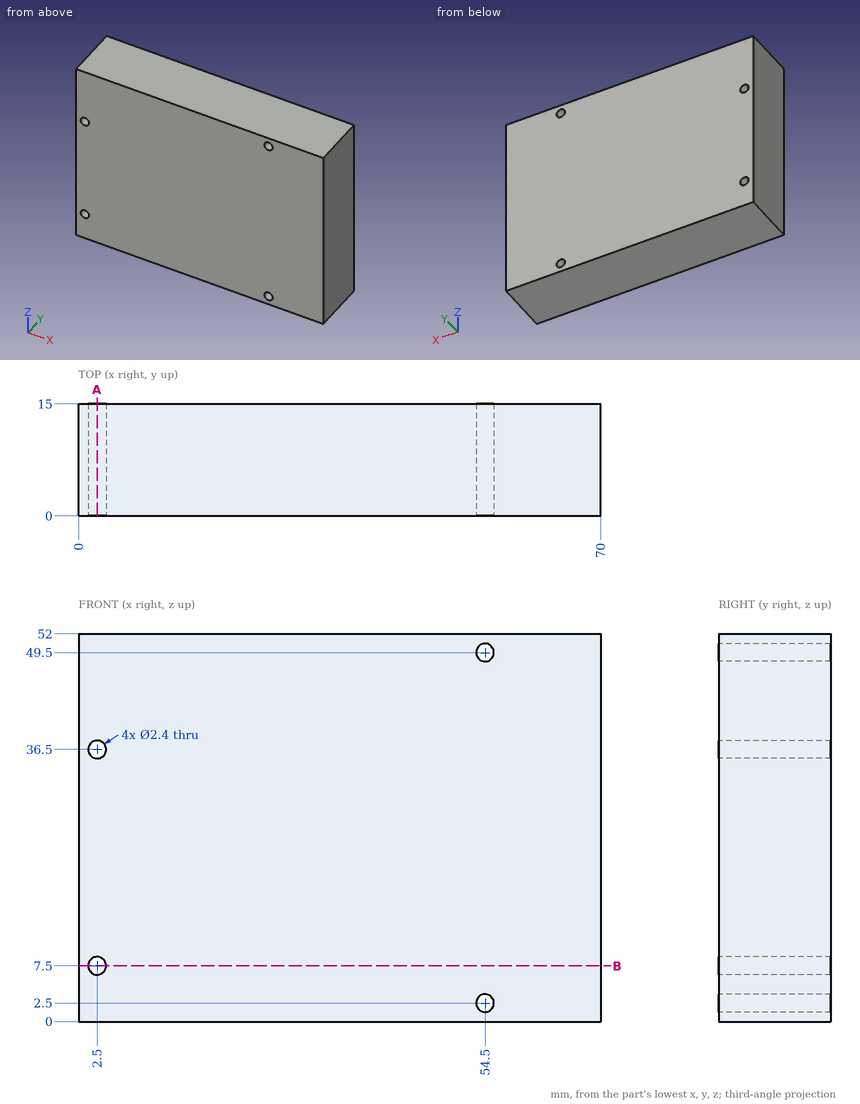
Answer from the drawing. Dimensions are ordinates in mm from the lowest x, y and z of the part. Give positions to 0.01 mm unless a question says otherwise; leave off trailing zeros. Loops run counter-clockwise (first coordinate to the right, second up) from the corner with the lowest first, then second, coordinate; pieces in that order, holes last. Notation, with made-up numbers: (84.25, 37) - (125.25, 37) arc R30 ccw to (125.25, 64) - close; hole circle Ø7 at (10, 35). An arc over 180 degrees is marked (long way). Answer as a JSON object with one key per item and string values.
1. A cutting plane is placed at A-A (x = 2.5). Write down the section's boundary in (y, z).
Determined:
{"outline": "(0, 0) - (15, 0) - (15, 6.3) - (0, 6.3) - close; (0, 8.7) - (15, 8.7) - (15, 35.3) - (0, 35.3) - close; (0, 37.7) - (15, 37.7) - (15, 52) - (0, 52) - close"}
2. A flat-ended cylindrical pin translates along its axis: pin 1 Ø1.9 at (x, z) = (54.5, 49.5) entering from +Y. Find the tip coordinate at first contact, or state that the pin passes through.
Determined:
{"pin 1": "through"}
3. Find the intervals of material crossed by L1, parallel to Z at x = 2.5, y = 7; L2, parallel to Z at x = 54.5, y = 5.5; L3, parallel to X at y = 11, z = 7.5, in increasing order. Write a range as [from, to].
Determined:
{"L1": "[0, 6.3], [8.7, 35.3], [37.7, 52]", "L2": "[0, 1.3], [3.7, 48.3], [50.7, 52]", "L3": "[0, 1.3], [3.7, 70]"}
4. A cutting plane is placed at B-B (z = 7.5). Write down the section's boundary in (x, y).
Determined:
{"outline": "(0, 0) - (1.3, 0) - (1.3, 15) - (0, 15) - close; (3.7, 0) - (70, 0) - (70, 15) - (3.7, 15) - close"}
